The model under review builds one solid part; all positions refer to its coordinate system, in mm. A direction names the side the tool comes from. Round coordinates to 2 decimals unless told otherwise and drop trailing zeros. Write each loop counter-clockwise with the first axis right and the second up, starting at its lowest first coordinate (ties: lowest second). Pieces come first, ordered by that corner, then holes. Notation, with made-up numbers: (71.25, 47) -> (96.25, 47) arc R30 cw to (96.25, 73) -> close; hole circle Ø11 at (24.5, 21.5). An arc over 180 degrees is marked (long way). Answer in a Markdown table with one row per item. Add a question column.
```python
from build123d import *

# Parameters (mm, degrees)
F0_W      = 701
F0_H      = 553
F1_DEPTH  = 15
F3_DEPTH  = 115
F5_D      = 10
F6_W      = 130
F6_H      = 553
F6_R      = 5
F7_DEPTH  = 369
F8_W      = 354
F8_H      = 113
F8_H_2    = 190
F9_DEPTH  = 115
F10_W     = 1070
F10_H     = 130
F11_DEPTH = 18
F12_W     = 635
F12_H     = 15
F13_DEPTH = 100
F15_D     = 8


with BuildPart() as f1:
    # F0 (on Front) → F1 (new body)
    with BuildSketch(Plane.XZ):
        with Locations((350.5, 276.5)):
            Rectangle(F0_W, F0_H)
    extrude(amount=-F1_DEPTH)

    # F2 (on face) → F3 (join)
    with BuildSketch(Plane.XZ):
        Polygon((0, 553), (0, 0), (15, 0), (15, 538), (686, 538), (686, 0), (701, 0), (701, 553), align=None)
    extrude(amount=F3_DEPTH)

    # F5 (through all)
    with Locations(Plane(origin=(0, 0, 0), x_dir=(0, -1, 0), z_dir=(-1, 0, 0))):
        with Locations((57.5, 57.5)):
            Hole(F5_D / 2)

    # F6 (on face) → F7 (join)
    with BuildSketch(Plane.YZ.offset(701)):
        with Locations((-50, 276.5)):
            Rectangle(F6_W, F6_H)
        with Locations((-57.5, 57.5)):
            Circle(F6_R, mode=Mode.SUBTRACT)
    extrude(amount=F7_DEPTH)

    # F8 (on face) → F9 (cut, through all)
    with BuildSketch(Plane.XZ.offset(115)):
        with Locations((878, 481.5)):
            Rectangle(F8_W, F8_H)
        with Locations((878, 315)):
            Rectangle(F8_W, F8_H_2)
        with Locations((878, 110)):
            Rectangle(F8_W, F8_H_2)
    extrude(amount=-F9_DEPTH, mode=Mode.SUBTRACT)

    # F10 (on face) → F11 (cut)
    with BuildSketch(Plane.XY.offset(553)):
        with Locations((535, -50)):
            Rectangle(F10_W, F10_H)
    extrude(amount=-F11_DEPTH, mode=Mode.SUBTRACT)

    # F12 (on face) → F13 (cut)
    with BuildSketch(Plane(origin=(0, 0, 0), x_dir=(1, 0, 0), z_dir=(0, 0, -1))):
        with Locations((350.5, -7.5)):
            Rectangle(F12_W, F12_H)
    extrude(amount=-F13_DEPTH, mode=Mode.SUBTRACT)

    # F15 (through all)
    with Locations(Plane(origin=(0, 15, 0), x_dir=(-1, 0, 0), z_dir=(0, 1, 0))):
        with Locations((-649, 345)):
            Hole(F15_D / 2)


solid = f1.part
```
1. Mouldability with a two-part tool opening along Z and no side actions: class faces 6 (the flat face through (572, 3, 535)), 7 (the flat face through (876, 0, 316)), 8 (the flat face through (9, -51, 0)) as pulls with the +Z half, pulls with the -Z half, needs draft (parallel to the pull), parting line crosses it, or undercut.
2. Tool access review of faces 1 (the flat face through (876, 0, 111)), 2 (the flat face through (15, -57, 264)), 3 (the flat face through (1070, -51, 271)), 4 (the flat face through (877, -115, 207)), 5 (the flat face through (876, -58, 425)): name each direction out of +Z, -Z, +X, -X, +Y, -Y from which nothing blocks a thin tool from reaching the whole face with its end or side.
3. For L1, parallel to Z at x = 785, y = -80; L2, parallel to X at y = -62, z = 190.5; L3, parallel to Y at x = 689, z = 57, list the stretches that pass through material, from the lowest coordinate up.
4. Add section D-D on x = 261. Write out the cut boundary in (y, z).
5. Add section B-B on x = 789. Write out the cut boundary in (y, z).
6. Insertion check: pin 1 Ø6 at (y, z) = (-26.5, 416.5) entering from -X; pin 2 Ø12 at (x, y) = (273.5, 11) entering from -Z; pin 3 Ø10 at (x, z) = (280.5, 442.5) entering from -Y. Each pin has a flat end and moves straight along its axis. Give the tip position at first contact, or say it passes through.
7. Add section A-A on y = -21. Write out the cut boundary in (x, z), plus the area to 3 significant figures.
8. Add section C-C on z = 144.5. Write out the cut boundary in (x, y).
Filled in:
| question | item | result |
|---|---|---|
| 1 | face 6 | pulls with the +Z half |
| 1 | face 7 | undercut |
| 1 | face 8 | pulls with the -Z half |
| 2 | face 1 | -Y |
| 2 | face 2 | +Z, -Z, -Y |
| 2 | face 3 | +Z, -Z, +X, +Y, -Y |
| 2 | face 4 | +Z, -Z, +X, -X, -Y |
| 2 | face 5 | +Z, -Y |
| 3 | L1 | 0 to 15, 205 to 220, 410 to 425 |
| 3 | L2 | 0 to 15, 686 to 701, 1055 to 1070 |
| 3 | L3 | -115 to -62.47, -52.53 to 15 |
| 4 | outline | (0, 100) -> (15, 100) -> (15, 535) -> (0, 535) -> close |
| 5 | outline | (-115, 0) -> (15, 0) -> (15, 535) -> (0, 535) -> (0, 425) -> (-115, 425) -> (-115, 410) -> (0, 410) -> (0, 220) -> (-115, 220) -> (-115, 205) -> (0, 205) -> (0, 15) -> (-115, 15) -> close |
| 6 | pin 1 | x = 0 |
| 6 | pin 2 | z = 100 |
| 6 | pin 3 | y = 0 |
| 7 | outline | (0, 0) -> (15, 0) -> (15, 535) -> (0, 535) -> close; (686, 0) -> (1070, 0) -> (1070, 535) -> (1055, 535) -> (1055, 425) -> (701, 425) -> (701, 535) -> (686, 535) -> close; hole (701, 15) -> (1055, 15) -> (1055, 205) -> (701, 205) -> close; hole (701, 220) -> (1055, 220) -> (1055, 410) -> (701, 410) -> close |
| 7 | area | 40,000 mm² |
| 8 | outline | (0, -115) -> (15, -115) -> (15, 0) -> (686, 0) -> (686, -115) -> (701, -115) -> (701, 0) -> (1055, 0) -> (1055, -115) -> (1070, -115) -> (1070, 15) -> (0, 15) -> close |
